Autodesk Inventor part; units mm, degrees
ref_plane "YZ Plane" through (0, 0, 0) normal (1, 0, 0) x (0, 1, 0)
ref_plane "XZ Plane" through (0, 0, 0) normal (0, 1, 0) x (-1, 0, 0)
ref_plane "XY Plane" through (0, 0, 0) normal (0, 0, 1) x (1, 0, 0)
sketch "Sketch1" plane through (0, 0, 0) normal (0, 1, 0) x (-1, 0, 0)
  line L0 (0, 0) -> (-76.2, 0)
  line L1 (-76.2, 0) -> (-76.2, -127)
  line L2 (-76.2, -127) -> (0, -127)
  line L3 (0, -127) -> (0, 0)
  dimension "d0" = 76.2
  dimension "d1" = 127
extrude "Extrusion1" add sketch "Sketch1" along normal blind 5.08
fillet "Fillet1" radius 38.1 2 edges at (76.2, 2.54, 0) (0, 2.54, 0)
sketch "Sketch2" plane through (0, 5.08, 0) normal (0, 1, 0) x (1, 0, 0)
  arc A0 (0, 38.1) -> (76.2, 38.1) centre (38.1, 38.1) ccw
  line L0 (38.1, 0) -> (38.1, 38.1)
  circle A1 centre (38.1, 38.1) radius 7.62
  circle A2 centre (38.1, 38.1) radius 5.08
  point P0 (0, 0)
  dimension "d5" = 15.24
  dimension "d6" = 10.16
extrude "Extrusion2" add sketch "Sketch2" along normal blind 5.08
properties part number "daodwaw"
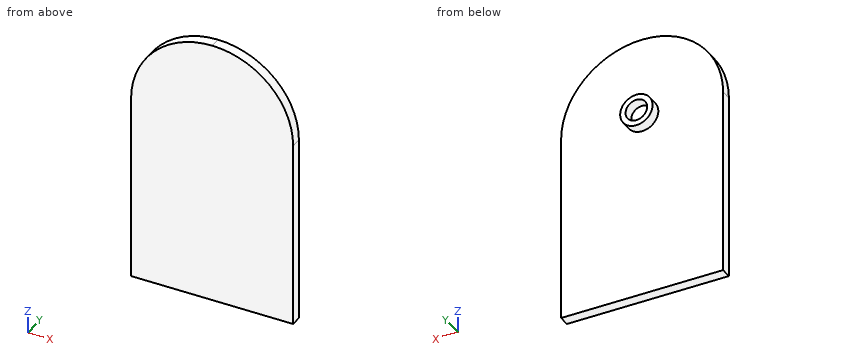
Could you check a few things on this model? Use its own coordinates, in mm. Give positions to 0.01 mm unless a question says otherwise; leave off trailing zeros. Write each loop counter-clockwise with the first axis right and the second up, starting at its lowest first coordinate (ties: lowest second). Pieces come first, ordered by that corner, then holes. Notation, with made-up numbers: (78, 51.5) - (119, 51.5) arc R36 cw to (119, 88.5) - close; hole circle Ø6 at (-33, -14). An arc over 180 degrees is marked (long way). One line per item, written item: value. Start each with the question number.
Item 1: Imagine slicing it at C-C, the plane x = 65.5. List the corners of the cut face in (y, z) for me, and give its area (3 significant figures).
Item 2: Imagine slicing it at A-A, the plane y = 6.75. List the corners of the cut face in (x, z) for me, and give its area (3 significant figures).
Item 3: I'm going to push flat-ended pins straight in: pin 1 (6 mm diameter, centred on x = 38.1, z = -38.1, fed in from +Y); pin 2 (3 mm diameter, centred on x = 28.5, z = -19, fed in from -Y); pin 3 (3 mm diameter, centred on x = 14.5, y = 8.5, fed in from -Z); pin 4 (2 mm diameter, centred on x = 34.5, y = 7, fed in from -Z). Where does each tip first touch, or does it pass through?
Item 4: Imagine slicing it at B-B, the plane z = -101. List the corners of the cut face in (x, y) for me.
Item 5: Please list where these lines run through material, in increasing order: line 1 (Z direction, x = 38.1, y = 8.9); line 2 (Y direction, x = 6, z = -52.5); line 3 (Z direction, x = 39.5, y = 1.25). Write a range as from..to.
Geometry says:
1. outline: (0, -127) - (5.08, -127) - (5.08, -11.63) - (0, -11.63) - close
1. area: 586 mm^2
2. outline: circle Ø15.24 at (38.1, -38.1); hole circle Ø10.16 at (38.1, -38.1)
2. area: 101 mm^2
3. pin 1: y = 5.08
3. pin 2: y = 0
3. pin 3: through
3. pin 4: z = -45.26
4. outline: (0, 0) - (76.2, 0) - (76.2, 5.08) - (0, 5.08) - close
5. line 1: -45.72..-43.18, -33.02..-30.48
5. line 2: 0..5.08
5. line 3: -127..-0.03
